```python
from build123d import *

# Parameters (mm, degrees)
BOSS_EXTRUDE1_DEPTH = 21
SHELL2_T            = -3
SKETCH2_W           = 34
SKETCH2_H           = 18
CUT_EXTRUDE1_DEPTH  = 3
FILLET2_R           = 2
SKETCH4_R           = 1.5
BOSS_EXTRUDE2_DEPTH = 3
CHAMFER1_SIZE       = 1


with BuildPart() as part:
    # Sketch1 → Boss-Extrude1 (new body)
    with BuildSketch(Plane(origin=(0, 0, 0), x_dir=(1, 0, 0), z_dir=(0, 1, 0))):
        Polygon((0, 54), (0, 0), (54, 0), (54, 54), (48, 54), (48, 58), (6, 58), (6, 54), align=None)
    extrude(amount=BOSS_EXTRUDE1_DEPTH)

    # Shell2
    shell2_openings = [part.faces().sort_by_distance(p)[0] for p in [
        (27, 21, -28.579766537),
    ]]
    offset(amount=SHELL2_T, openings=shell2_openings, kind=Kind.INTERSECTION)

    # Sketch2 → Cut-Extrude1 (cut)
    with BuildSketch(Plane(origin=(0, 0, -58), x_dir=(-1, 0, 0), z_dir=(0, 0, -1))):
        with Locations((-27, 12)):
            Rectangle(SKETCH2_W, SKETCH2_H)
    extrude(amount=-CUT_EXTRUDE1_DEPTH, mode=Mode.SUBTRACT)

    # Fillet2
    fillet2_edges = [part.edges().sort_by_distance(p)[0] for p in [
        (6, 10.5, -58),
        (6, 10.5, -54),
        (0, 10.5, -54),
        (0, 10.5, 0),
        (54, 10.5, 0),
        (48, 10.5, -54),
        (48, 10.5, -58),
        (54, 10.5, -54),
    ]]
    fillet(fillet2_edges, radius=FILLET2_R - 0.0001)  # a hair under: the kernel refuses the full size

    # Sketch4 → Boss-Extrude2 (add)
    # profile 1 of 4: a face of its own
    with BuildSketch(Plane(origin=(0, 21, 0), x_dir=(1, 0, 0), z_dir=(0, 1, 0))):
        with BuildLine():
            Line((0, 51), (0, 45))
            Line((0, 45), (-4, 45))
            ThreePointArc((-4, 45), (-7, 48), (-4, 51))
            Line((-4, 51), (0, 51))
        make_face()
        with Locations(Location((-4, 48, 0), (0, 0, 270))):
            Circle(SKETCH4_R, mode=Mode.SUBTRACT)
    # profile 2 of 4: a face of its own
    with BuildSketch(Plane(origin=(0, 21, 0), x_dir=(1, 0, 0), z_dir=(0, 1, 0))):
        with BuildLine():
            Line((-4, 3), (0, 3))
            Line((0, 3), (0, 9))
            Line((0, 9), (-4, 9))
            ThreePointArc((-4, 9), (-7, 6), (-4, 3))
        make_face()
        with Locations(Location((-4, 6, 0), (0, 0, 90))):
            Circle(SKETCH4_R, mode=Mode.SUBTRACT)
    # profile 3 of 4: a face of its own
    with BuildSketch(Plane(origin=(0, 21, 0), x_dir=(1, 0, 0), z_dir=(0, 1, 0))):
        with BuildLine():
            Line((58, 9), (54, 9))
            Line((54, 9), (54, 3))
            Line((54, 3), (58, 3))
            ThreePointArc((58, 3), (61, 6), (58, 9))
        make_face()
        with Locations(Location((58, 6, 0), (0, 0, 270))):
            Circle(SKETCH4_R, mode=Mode.SUBTRACT)
    # profile 4 of 4: a face of its own
    with BuildSketch(Plane(origin=(0, 21, 0), x_dir=(1, 0, 0), z_dir=(0, 1, 0))):
        with BuildLine():
            Line((58, 51), (54, 51))
            Line((54, 51), (54, 45))
            Line((54, 45), (58, 45))
            ThreePointArc((58, 45), (61, 48), (58, 51))
        make_face()
        with Locations(Location((58, 48, 0), (0, 0, 90))):
            Circle(SKETCH4_R, mode=Mode.SUBTRACT)
    extrude(amount=-BOSS_EXTRUDE2_DEPTH)

    # Chamfer1
    chamfer1_edges = [part.edges().sort_by_distance(p)[0] for p in [
        (-4, 18, -49.5),
        (-4, 18, -4.5),
        (58, 18, -7.5),
        (58, 18, -46.5),
    ]]
    chamfer(chamfer1_edges, length=CHAMFER1_SIZE)


solid = part.part
```
For this review, take the finished solid that the model builds, in its own axes (mm). A direction names the side the tool comes from. Round coordinates to 2 decimals unless told otherwise and drop trailing zeros. Loops run counter-clockwise (first coordinate to the right, second up) from the corner with the lowest first, then second, coordinate; pieces in that order, holes last.
Q1. Add section B-B on z = -20. Write out the cut boundary in (x, y).
Result sheet:
outline: (0, 0) - (54, 0) - (54, 21) - (51, 21) - (51, 3) - (3, 3) - (3, 21) - (0, 21) - close
Q2. Insertion check: pin 1 Ø5 at (x, z) = (57, -47.5) entering from -Y; pin 2 Ø12 at (y, z) = (5, -50) entering from +X; pin 3 Ø2 at (x, y) = (15.5, 14.5) entering from -Z. Each pin has a flat end and moves straight along its axis. Give the tip position at first contact, or say it passes through.
Result sheet:
pin 1: stops at y = 18
pin 2: stops at x = 54
pin 3: stops at z = -3
Q3. Machinability: for faces 4 (the face through (56, 20, -9)), 5 (the face through (56, 20, -51)), 6 (the face through (-1, 18, -6)), 7 (the face through (3, 10, -54)), 8 (the face through (6, 12, -51)), which of the approach directions +Z, -Z, +X, -X, +Y, -Y give a long, thin tool a straight path to every point of the face, cutting with its end or side? Answer none if there is none.
Result sheet:
face 4: +X, +Y, -Y
face 5: -Z, +X, +Y, -Y
face 6: +Z, -Z, -X, -Y
face 7: -Z, -X, +Y, -Y
face 8: +Y
Q4. Mouldability with a two-part tool opening along X and no side actions: class faces 1 (the face through (53.4, 10.65, -0.57)), 2 (the face through (-2, 20, -45)), 3 (the face through (9, 12, -53)) as +X half, -X half, draft (parallel to the pull), parting line (faces both ways), or undercut.
Result sheet:
face 1: +X half
face 2: draft
face 3: undercut
Q5. Add section A-A on z = -48. Write out the cut boundary in (x, y).
Result sheet:
outline: (-7, 18) - (-6.5, 18) - (-5.5, 19) - (-5.5, 21) - (-7, 21) - close; (-2.5, 19) - (-1.5, 18) - (0, 18) - (0, 0) - (54, 0) - (54, 18) - (55.5, 18) - (56.5, 19) - (56.5, 21) - (51, 21) - (51, 3) - (3, 3) - (3, 21) - (-2.5, 21) - close; (59.5, 19) - (60.5, 18) - (61, 18) - (61, 21) - (59.5, 21) - close
Q6. To check wall thickness, follow line 1 along X through (y, z) = (19.55, -6); line 2 along X through (y, z) = (7, -37.5); line 3 along Z through (x, y) = (23.5, 4.75). State the ranges of each line that lie inside material, in increasing order.
Result sheet:
line 1: x = -7 to -5.5, -2.5 to 3, 51 to 56.5, 59.5 to 61
line 2: x = 0 to 3, 51 to 54
line 3: z = -3 to 0
Q7. Add section D-D on x = 43. Write out the cut boundary in (y, z), plus the area to 3 significant figures.
Result sheet:
outline: (0, -58) - (3, -58) - (3, -3) - (21, -3) - (21, 0) - (0, 0) - close
area: 228 mm2
